Geometry check sheet. Reference: the model listing, model coordinates, mm. Round coordinates to 2 decimals unless told otherwise and drop trailing zeros. Write each loop counter-clockwise with the first axis right and the second up, starting at its lowest first coordinate (ties: lowest second). Pieces come first, ordered by that corner, then holes. Notation, with made-up numbers: M 60.25,-17.75 L 105.25,-17.75 A4 ccw 105.25,-12.75 Z; hole C 62.25,20.5 d7. An arc over 180 degrees is marked long. Use a Markdown table: item, result.
Autodesk Inventor part; units mm, degrees
ref_plane "YZ Plane" through (0, 0, 0) normal (1, 0, 0) x (0, 1, 0)
ref_plane "XZ Plane" through (0, 0, 0) normal (0, 1, 0) x (-1, 0, 0)
ref_plane "XY Plane" through (0, 0, 0) normal (0, 0, 1) x (1, 0, 0)
sketch "スケッチ1" plane through (0, 0, 0) normal (0, 0, 1) x (1, 0, 0)
  circle A0 centre (0, 0) radius 47.5
  circle A1 centre (0, 0) radius 67.5
  dimension "d0" = 95
  dimension "d1" = 135
extrude "押し出し1" add sketch "スケッチ1" along normal blind 10
sketch "スケッチ2" plane through (0, 0, 10) normal (0, 0, 1) x (1, 0, 0)
  circle A0 centre (0, 0) radius 62.5
  point P0 (16.1762, 60.3704)
  point P1 (-16.1762, 60.3704)
  point P2 (-44.1942, 44.1942)
  point P3 (-60.3704, 16.1762)
  point P4 (-60.3704, -16.1762)
  point P5 (-44.1942, -44.1942)
  point P6 (-16.1762, -60.3704)
  point P7 (16.1762, -60.3704)
  point P8 (44.1942, -44.1942)
  point P9 (60.3704, -16.1762)
  point P10 (60.3704, 16.1762)
  point P11 (44.1942, 44.1942)
  dimension "d4" = 125
  dimension "d7" = 360
  dimension "d25" = 0
hole "穴1" at (16.1762, 60.3704, 10) at (-16.1762, 60.3704, 10) at (-44.1942, 44.1942, 10) at (-60.3704, 16.1762, 10) at (-60.3704, -16.1762, 10) at (-44.1942, -44.1942, 10) at (-16.1762, -60.3704, 10) at (16.1762, -60.3704, 10) at (44.1942, -44.1942, 10) at (60.3704, -16.1762, 10) at (60.3704, 16.1762, 10) at (44.1942, 44.1942, 10) direction (0, 0, -1) diameter 4.5 end through all
chamfer "面取り1" distance 1 angle 45 2 edges at (-47.5, 0, 10) (-47.5, 0, 0)
sketch "スケッチ3" plane through (0, 0, 10) normal (0, 0, 1) x (1, 0, 0)
  circle A0 centre (16.1762, 60.3704) radius 2.25
  circle A1 centre (-16.1762, 60.3704) radius 2.25
  circle A2 centre (0, 0) radius 67.5
  circle A3 centre (0, 0) radius 62.5
  circle A4 centre (-16.1762, 60.3704) radius 5
  circle A5 centre (16.1762, 60.3704) radius 5
  point P0 (11.2987, 61.4702)
  point P1 (17.4703, 65.2)
  point P2 (-17.4703, 65.2)
  point P3 (-20.9502, 58.8841)
properties part number "unit-j2-base2" material "ABS プラスチック"
Item 1: Go/stop test with flat-tipped pins: pin 1 (4 mm diameter, centred on y = -23.5, z = 4.5, fed in from +X); pin 2 (1.5 mm diameter, centred on x = 22.5, z = 4.5, fed in from +Y); pin 3 (3 mm diameter, centred on x = -6, z = 6, fed in from -Y). Record where each tip stops, or that it passes through.
Outcome:
| item | result |
|---|---|
| pin 1 | stops at x = 63.98 |
| pin 2 | stops at y = 63.9 |
| pin 3 | stops at y = -67.35 |
Item 2: Mould release check, pull along Y, two halves, no side actions. Record for faces 1 (the face through (-53.57, 41.07, 4.93)), 2 (the face through (45, 20, 0)), 3 (the face through (-16.852, 58.224, 4.93)): +Y half, -Y half, draft (parallel to the pull), parting line (faces both ways), or undercut.
Outcome:
| item | result |
|---|---|
| face 1 | parting line |
| face 2 | draft |
| face 3 | undercut |
Item 3: Cross-section at C-C, the plane z = 4.75. Count the separate pieces of the cut face and the enclosed holes in it, and give its area (3 significant figures).
Outcome:
| item | result |
|---|---|
| separate pieces | 1 |
| enclosed holes | 13 |
| area | 7,030 mm2 |
Item 4: Material ranges on line 1 along X through (y, z) = (-44, 6.5); line 2 along Y through (x, z) = (-17.5, 8); line 3 along Y through (x, z) = (1.5, 8.25), recorded low to high. Write a range as from..to.
Outcome:
| item | result |
|---|---|
| line 1 | x = -51.19..-46.44, -41.95..-17.9, 17.9..41.95, 46.44..51.19 |
| line 2 | y = -65.19..-62.19, -58.55..-44.16, 44.16..58.55, 62.19..65.19 |
| line 3 | y = -67.48..-47.48, 47.48..67.48 |
Item 5: Cross-section at A-A, the plane x = 0. Record the cut outline in (y, z).
Outcome:
| item | result |
|---|---|
| outline | M -67.5,0 L -48.5,0 L -47.5,1 L -47.5,9 L -48.5,10 L -67.5,10 Z; M 47.5,1 L 48.5,0 L 67.5,0 L 67.5,10 L 48.5,10 L 47.5,9 Z |
